from build123d import *

# Parameters (mm, degrees)
BOSS_EXTRUDE1_DEPTH = 89
SKETCH2_R           = 2
CUT_EXTRUDE1_DEPTH  = 26
BOSS_EXTRUDE2_DEPTH = 89
SKETCH4_W           = 47.922407602
SKETCH4_H           = 26.699627092
BOSS_EXTRUDE3_DEPTH = 20
SKETCH7_R           = 2.5
CUT_EXTRUDE2_DEPTH  = 299.356682512
SKETCH9_W           = 15
SKETCH9_H           = 8
CUT_EXTRUDE3_DEPTH  = 305.5939264
CUT_EXTRUDE4_REACH  = 304.791
SKETCH8_R           = 2.5


with BuildPart() as part:
    # Sketch1 → Boss-Extrude1 (new body)
    with BuildSketch(Plane.XY):
        Polygon((-283, 0), (0, 0), (0, 15), (-217.53, 15), (-217.53, 11), (-237.53, 11), (-237.53, 15), (-254.5, 15), (-254.5, 11), (-274, 11), (-274, 15), (-283, 15), align=None)
    extrude(amount=BOSS_EXTRUDE1_DEPTH)

    # Sketch2 → Cut-Extrude1 (cut)
    with BuildSketch(Plane(origin=(0, 15, 0), x_dir=(1, 0, 0), z_dir=(0, 1, 0))):
        with Locations(Location((-246.015, -44.5, 0), (0, 0, 180))):
            Circle(SKETCH2_R)
    extrude(amount=-CUT_EXTRUDE1_DEPTH, mode=Mode.SUBTRACT)

    # Sketch3 → Boss-Extrude2 (add)
    with BuildSketch(Plane(origin=(0, 0, 0), x_dir=(-1, 0, 0), z_dir=(0, 0, -1))):
        Polygon((0, 0), (0, -61.6), (0, -69.046795722), (18.017528485, -69.046795722), (26.551464217, -45.6), (53.448535783, -45.6), (61.982471515, -69.046795722), (138.017528485, -69.046795722), (146.551464217, -45.6), (173.448535783, -45.6), (181.982471515, -69.046795722), (200, -69.046795722), (200, -61.6), (200, 7.5), (0, 7.5), align=None)
    extrude(amount=-BOSS_EXTRUDE2_DEPTH)

    # Sketch4 → Boss-Extrude3 (add, symmetric)
    with BuildSketch(Plane(origin=(0, 0, 44.5), x_dir=(-1, 0, 0), z_dir=(0, 0, -1))):
        with Locations((40.197751444, -51.696982176)):
            Rectangle(SKETCH4_W, SKETCH4_H)
    extrude(amount=BOSS_EXTRUDE3_DEPTH, both=True)

    # Sketch7 → Cut-Extrude2 (cut, through all)
    with BuildSketch(Plane(origin=(0, 0, 24.5), x_dir=(-1, 0, 0), z_dir=(0, 0, -1))):
        with Locations((40, -61.6)):
            Circle(SKETCH7_R)
    extrude(amount=-CUT_EXTRUDE2_DEPTH, mode=Mode.SUBTRACT)

    # Sketch9 → Cut-Extrude3 (cut, through all)
    with BuildSketch(Plane(origin=(0, 0, 0), x_dir=(-1, 0, 0), z_dir=(0, 0, -1))):
        with Locations((160, -36.6)):
            Rectangle(SKETCH9_W, SKETCH9_H)
    extrude(amount=-CUT_EXTRUDE3_DEPTH, mode=Mode.SUBTRACT)

    # Sketch8 → Cut-Extrude4 (cut, up to next)
    with BuildSketch(Plane.XZ.offset(45.6), mode=Mode.PRIVATE) as cut_extrude4_sk1:
        with Locations(Location((-160, 74, 0), (0, 0, 270))):
            Circle(SKETCH8_R)
    cut_extrude4_tool1 = extrude(cut_extrude4_sk1.sketch, amount=-CUT_EXTRUDE4_REACH, mode=Mode.PRIVATE) & part.part
    # Sketch8 → Cut-Extrude4 (cut, up to next)
    with BuildSketch(Plane.XZ.offset(45.6), mode=Mode.PRIVATE) as cut_extrude4_sk2:
        with Locations(Location((-160, 15, 0), (0, 0, 270))):
            Circle(SKETCH8_R)
    cut_extrude4_tool2 = extrude(cut_extrude4_sk2.sketch, amount=-CUT_EXTRUDE4_REACH, mode=Mode.PRIVATE) & part.part
    add(cut_extrude4_tool1.solids().sort_by_distance((-160, -45.6, 74))[0], mode=Mode.SUBTRACT)
    add(cut_extrude4_tool2.solids().sort_by_distance((-160, -45.6, 15))[0], mode=Mode.SUBTRACT)


solid = part.part
For this review, take the finished solid that the model builds, in its own axes (mm). A direction names the side the tool comes from. Round coordinates to 2 decimals unless told otherwise and drop trailing zeros. Order: outer loops, then holes, each group sorted by start corner. A loop starts at its lowest first (then second) coordinate and runs counter-clockwise, first axis right, second up. Notation, with made-up numbers: M 78,-2.5 L 129,-2.5 A23 cw 129,31.5 Z; hole C 0,57 d5. An arc over 180 degrees is marked long. Use a Markdown table: item, result. Add a question column.
Item 1: To check wall thickness, follow line 1 along Z through (x, y) = (-160, -43); line 2 along X through (y, z) = (-33.5, 21); line 3 along X through (y, z) = (-44.55, 15). State the ranges of each line that lie inside material, in increasing order.
Item 2: Add section D-D, the plane y = -51. Give the boundary of the cut face in (x, z).
Item 3: Add section C-C, the plane x = -40. Give the boundary of the cut face in (y, z).
Item 4: Add section B-B, the plane z = 20. Give the boundary of the cut face in (x, y), then the cut area to 3 significant figures.
Item 5: Add section A-A, the plane x = -160. Give the boundary of the cut face in (y, z).
Item 6: Insertion check: pin 1 (6 mm diameter, centred on x = -160, z = 15, fed in from -Y); pin 2 (1 mm diameter, centred on y = -17, z = 31, fed in from -X); pin 3 (2 mm diameter, centred on x = -43.5, z = 36, fed in from -Y); pin 4 (3 mm diameter, centred on x = -40, y = -61.6, fed in from +Z). Each pin has a flat end and moves straight along its axis. Give the tip position at first contact, or say it passes through.
Item 7: Tool access review of faces 4 (the flat face through (-177.656, -57.159, 43.877)), 5 (the flat face through (-200, -35, 44)), 6 (the flat face through (-160, -32.6, 44)), 7 (the flat face through (-40, -55, 64.5)): name each direction out of +Z, -Z, +X, -X, +Y, -Y from which nothing blocks a thin tool from reaching the whole face with its end or side.
Item 8: Mouldability with a two-part tool opening along X and no side actions: class faces 1 (the flat face through (-283, 8, 44)), 2 (the flat face through (-160, -45.6, 44)), 3 (the flat face through (-191, -69.047, 44)) as released by +X, released by -X, zero draft, split by the parting line, or undercut.
Geometry results:
| question | item | result |
|---|---|---|
| 1 | line 1 | z = 0 to 12.5, 17.5 to 71.5, 76.5 to 89 |
| 1 | line 2 | x = -200 to -167.5, -152.5 to 0 |
| 1 | line 3 | x = -200 to -162.5, -157.5 to 0 |
| 2 | outline | M -200,0 L -175.41,0 L -175.41,89 L -200,89 Z; M -144.59,0 L -55.41,0 L -55.41,24.5 L -24.59,24.5 L -24.59,0 L 0,0 L 0,89 L -24.59,89 L -24.59,64.5 L -55.41,64.5 L -55.41,89 L -144.59,89 Z |
| 3 | outline | M -65.05,24.5 L -64.1,24.5 L -64.1,64.5 L -65.05,64.5 Z; M -59.1,24.5 L -45.6,24.5 L -45.6,0 L 15,0 L 15,89 L -45.6,89 L -45.6,64.5 L -59.1,64.5 Z |
| 4 | outline | M -283,0 L -200,0 L -200,-69.05 L -181.98,-69.05 L -173.45,-45.6 L -146.55,-45.6 L -138.02,-69.05 L -61.98,-69.05 L -53.45,-45.6 L -26.55,-45.6 L -18.02,-69.05 L 0,-69.05 L 0,15 L -217.53,15 L -217.53,11 L -237.53,11 L -237.53,15 L -254.5,15 L -254.5,11 L -274,11 L -274,15 L -283,15 Z; hole M -167.5,-40.6 L -152.5,-40.6 L -152.5,-32.6 L -167.5,-32.6 Z |
| 4 | area | 16,100 mm² |
| 5 | outline | M -45.6,0 L -40.6,0 L -40.6,12.5 L -45.6,12.5 Z; M -45.6,17.5 L -40.6,17.5 L -40.6,71.5 L -45.6,71.5 Z; M -45.6,76.5 L -40.6,76.5 L -40.6,89 L -45.6,89 Z; M -32.6,0 L 15,0 L 15,89 L -32.6,89 Z |
| 6 | pin 1 | stops at y = -45.6 |
| 6 | pin 2 | stops at x = -200 |
| 6 | pin 3 | stops at y = -65.05 |
| 6 | pin 4 | passes through |
| 7 | face 4 | +Z, -Z, -Y |
| 7 | face 5 | +Z, -Z, -X, -Y |
| 7 | face 6 | +Z, -Z |
| 7 | face 7 | +Z, -Y |
| 8 | face 1 | released by -X |
| 8 | face 2 | undercut |
| 8 | face 3 | zero draft |
